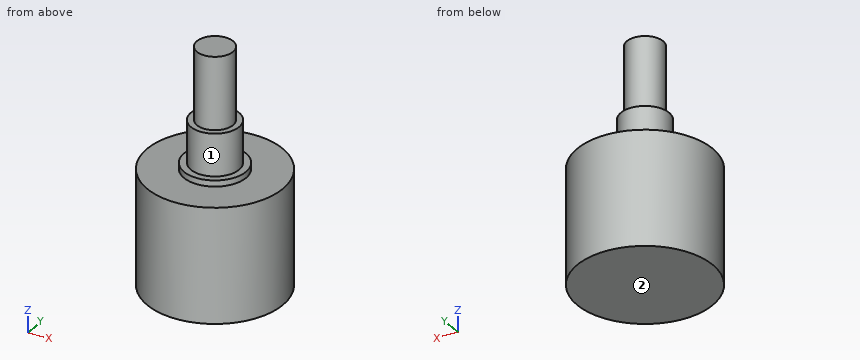
Autodesk Inventor part; units mm, degrees
ref_plane "YZ Plane" through (0, 0, 0) normal (1, 0, 0) x (0, 1, 0)
ref_plane "XZ Plane" through (0, 0, 0) normal (0, 1, 0) x (-1, 0, 0)
ref_plane "XY Plane" through (0, 0, 0) normal (0, 0, 1) x (1, 0, 0)
sketch "スケッチ1" plane through (0, 0, 0) normal (0, 0, 1) x (1, 0, 0)
  circle A0 centre (0, 0) radius 11.25
  dimension "d0" = 22.5
extrude "押し出し1" add sketch "スケッチ1" along normal blind 19
sketch "スケッチ2" plane through (0, 0, 19) normal (0, 0, 1) x (1, 0, 0)
  circle A0 centre (0, 0) radius 11.25
  circle A1 centre (0, 0) radius 5.15
  dimension "d3" = 10.3
extrude "押し出し2" add sketch "スケッチ2" along normal blind 1 contours A1
sketch "スケッチ3" plane through (0, 0, 20) normal (0, 0, 1) x (1, 0, 0)
  circle A0 centre (0, 0) radius 5.15
  circle A1 centre (0, 0) radius 4
  dimension "d6" = 8
extrude "押し出し3" add sketch "スケッチ3" along normal blind 7 contours A1
sketch "スケッチ4" plane through (0, 0, 27) normal (0, 0, 1) x (1, 0, 0)
  circle A0 centre (0, 0) radius 4
  circle A1 centre (0, 0) radius 3
  dimension "d9" = 6
extrude "押し出し4" add sketch "スケッチ4" along normal blind 12 contours A1
thread "ねじ1"
properties part number "ポテンションメーター_ＢＩ-７２８４_rev2"
The model under review builds one solid part; all positions refer to its coordinate system, in mm. Face numbers are marked on the shaded views. A direction names the side the tool comes from. Give positions to 0.01 mm unless a question says otherwise; leave off trailing zeros. Loops run counter-clockwise (first coordinate to the right, second up) from the corner with the lowest first, then second, coordinate; pieces in that order, holes last. Notation, with made-up numbers: (10.5, -13) -> (69.5, -13) arc R11 cw to (69.5, 8) -> close; hole circle Ø1 at (57, 33.5). An arc over 180 degrees is marked (long way). Answer as a JSON object with one key per item and string values. Group by question number.
Q1. Take a section at D-D (x = 8). Write out the cut boundary in (y, z).
Q2. Take a section at C-C (z = 21). Write out the cut boundary in (x, y).
Q3. Tool access review of the marked faces 1 and 2: name each direction out of +Z, -Z, +X, -X, +Y, -Y from which nothing blocks a thin tool from reaching the whole face with its end or side.
Q4. Take a section at A-A (x = 0). Write out the cut boundary in (y, z), plus the area to 3 significant figures.
Q5. Insertion check: pin 1 (8 mm diameter, centred on x = 6, y = -5.5, fed in from +Z); pin 2 (1.5 mm diameter, centred on x = -5.5, z = 12, fed in from +Y); pin 3 (1.5 mm diameter, centred on x = -2.5, y = 3, fed in from +Z). Each pin has a flat end and moves straight along its axis. Give the tip position at first contact, or say it passes through.
Q6. Wall thickness on line 1 along Z through (x, y) = (8.5, -5); line 2 along Z through (x, y) = (-3.75, 2.25); line 3 along X through (y, z) = (2.5, 10): over which ranges is each line inside the solid? List them lowest first.
Answer below:
{
 "1": {"outline": "(-7.91, 0) -> (7.91, 0) -> (7.91, 19) -> (-7.91, 19) -> close"},
 "2": {"outline": "circle Ø8 at (0, 0)"},
 "3": {"face 1": "+Z", "face 2": "-Z, +X, -X, +Y, -Y"},
 "4": {"outline": "(-11.25, 0) -> (11.25, 0) -> (11.25, 19) -> (5.15, 19) -> (5.15, 20) -> (4, 20) -> (4, 27) -> (3, 27) -> (3, 39) -> (-3, 39) -> (-3, 27) -> (-4, 27) -> (-4, 20) -> (-5.15, 20) -> (-5.15, 19) -> (-11.25, 19) -> close", "area": "566 mm2"},
 "5": {"pin 1": "stops at z = 20", "pin 2": "stops at y = 10.2", "pin 3": "stops at z = 27"},
 "6": {"line 1": "z = 0 to 19", "line 2": "z = 0 to 20", "line 3": "x = -10.97 to 10.97"}
}
